Model file for the job. Use its own axes, mm. Face numbers are marked on the shaded views. A direction names the side the tool comes from. Coordinates: 2 decimals unless noted, no trailing zeros. Order: outer loops, then holes, each group sorted by start corner. A loop starts at its lowest first (then second) coordinate and runs counter-clockwise, first axis right, second up.
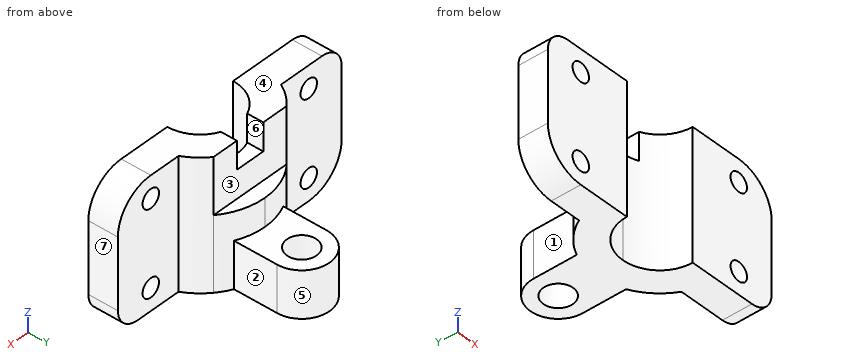
from build123d import *

# Parameters (mm, degrees)
EXTRUDE_1_DEPTH     = 70
CUT_EXTRUDE_2_DEPTH = 30
SKETCH_5_W          = 16
SKETCH_5_H          = 15
CUT_EXTRUDE_3_DEPTH = 102.257098517
EXTRUDE_START       = -25
SKETCH_6_R          = 8
EXTRUDE_2_DEPTH     = 25
SKETCH_7_R          = 5
CUT_EXTRUDE_4_DEPTH = 112.534747949
FILLET_1_R          = 20
FILLET_2_R          = 12


with BuildPart() as part:
    # Sketch 1 → Extrude 1 (new body)
    with BuildSketch(Plane.XY):
        with BuildLine():
            ThreePointArc((-20, 0), (-14.142135624, 14.142135624), (0, 20))
            Line((0, 20), (0, 27))
            Line((0, 27), (-22.271057451, 27))
            ThreePointArc((-22.271057451, 27), (-27.26050724, 21.951417836), (-31.128764833, 16))
            Line((-31.128764833, 16), (-68, 16))
            Line((-68, 16), (-68, 0))
            Line((-68, 0), (-20, 0))
        make_face()
        with BuildLine():
            Line((0, 27), (0, 20))
            ThreePointArc((0, 20), (14.142135624, 14.142135624), (20, 0))
            Line((20, 0), (68, 0))
            Line((68, 0), (68, 16))
            Line((68, 16), (31.128764833, 16))
            ThreePointArc((31.128764833, 16), (27.26050724, 21.951417836), (22.271057451, 27))
            Line((22.271057451, 27), (0, 27))
        make_face()
        with BuildLine():
            Line((-22.271057451, 27), (0, 27))
            Line((0, 27), (0, 35))
            ThreePointArc((0, 35), (-11.832159566, 32.939338184), (-22.271057451, 27))
        make_face()
        with BuildLine():
            Line((0, 35), (0, 27))
            Line((0, 27), (22.271057451, 27))
            ThreePointArc((22.271057451, 27), (11.832159566, 32.939338184), (0, 35))
        make_face()
    extrude(amount=-EXTRUDE_1_DEPTH)

    # Sketch 1_13 → Cut-Extrude 2 (cut)
    with BuildSketch(Plane.XY):
        with BuildLine():
            Line((-22.271057451, 27), (0, 27))
            Line((0, 27), (0, 35))
            ThreePointArc((0, 35), (-11.832159566, 32.939338184), (-22.271057451, 27))
        make_face()
        with BuildLine():
            Line((0, 35), (0, 27))
            Line((0, 27), (22.271057451, 27))
            ThreePointArc((22.271057451, 27), (11.832159566, 32.939338184), (0, 35))
        make_face()
    extrude(amount=-CUT_EXTRUDE_2_DEPTH, mode=Mode.SUBTRACT)

    # Sketch 5 → Cut-Extrude 3 (cut, through all)
    with BuildSketch(Plane(origin=(0, 27, 0), x_dir=(1, 0, 0), z_dir=(0, 1, 0))):
        with Locations((0, 7.5)):
            Rectangle(SKETCH_5_W, SKETCH_5_H)
    extrude(amount=-CUT_EXTRUDE_3_DEPTH, mode=Mode.SUBTRACT)

    # Sketch 6 → Extrude 2 (add)
    with BuildSketch(Plane(origin=(0, 0, -70), x_dir=(-1, 0, 0), z_dir=(0, 0, -1)).offset(EXTRUDE_START)):
        with BuildLine():
            Line((-15, 31.622776602), (-15, 55))
            ThreePointArc((-15, 55), (0, 70), (15, 55))
            Line((15, 55), (15, 31.622776602))
            ThreePointArc((15, 31.622776602), (0, 35), (-15, 31.622776602))
        make_face()
        with Locations((0, 55)):
            Circle(SKETCH_6_R, mode=Mode.SUBTRACT)
    extrude(amount=EXTRUDE_2_DEPTH)

    # Sketch 7 → Cut-Extrude 4 (cut, through all)
    with BuildSketch(Plane(origin=(0, 16, 0), x_dir=(1, 0, 0), z_dir=(0, 1, 0))):
        with Locations(Location((-48, 12, 0), (0, 0, 180))):
            Circle(SKETCH_7_R)
        with Locations((-48, 58)):
            Circle(SKETCH_7_R)
        with Locations(Location((48, 58, 0), (0, 0, 180))):
            Circle(SKETCH_7_R)
        with Locations((48, 12)):
            Circle(SKETCH_7_R)
    extrude(amount=-CUT_EXTRUDE_4_DEPTH, mode=Mode.SUBTRACT)

    # Fillet 1
    fillet_1_edges = [part.edges().sort_by_distance(p)[0] for p in [
        (68, 8, 0),
        (-68, 8, -70),
    ]]
    fillet(fillet_1_edges, radius=FILLET_1_R)

    # Fillet 2
    fillet_2_edges = [part.edges().sort_by_distance(p)[0] for p in [
        (-68, 8, 0),
        (68, 8, -70),
    ]]
    fillet(fillet_2_edges, radius=FILLET_2_R)


solid = part.part
Q1. Cut at B-B, the plane y = 24.5. List the corners of the cut face in (x, z) (3 decimals).
Established:
outline: (-24.995, -70) - (24.995, -70) - (24.995, 0) - (8, 0) - (8, -15) - (-8, -15) - (-8, 0) - (-24.995, 0) - close
Q2. Drop flat-ended pins along their axis: P1, Ø13, axis at x = 48, z = -12, coming from the +Y side; P2, Ø8, axis at x = -11, z = -29.5, coming from the +Y side; P3, Ø9, axis at x = 4, z = -9.5, coming from the +Y side; P4, Ø2, axis at x = -23.5, z = -26, coming from the -Y side. Give the stop position or say it passes through.
Established:
P1: stops at y = 16
P2: stops at y = 34.29
P3: stops at y = 27
P4: stops at y = 0
Q3. Cut at A-A, the plane y = 52. List the corners of the cut face in (x, z).
Established:
outline: (-15, -70) - (-7.42, -70) - (-7.42, -45) - (-15, -45) - close; (7.42, -70) - (15, -70) - (15, -45) - (7.42, -45) - close
Q4. Cut at D-D, the plane x = -25.5. List the corners of the cut face in (y, z), plus the area to 3 significant figures.
Established:
outline: (0, -70) - (23.97, -70) - (23.97, 0) - (0, 0) - close
area: 1,680 mm2
Q5. Mould opens along X. For the marked faces 4, 5, 6 and 7 say: pulls with the +X half, pulls with the -X half, needs draft (parallel to the pull), parting line crosses it, or undercut.
Established:
face 4: needs draft
face 5: parting line crosses it
face 6: undercut
face 7: pulls with the +X half
Q6. Cut at C-C, the plane x = 27. List the corners of the cut face in (y, z), plus the area to 3 significant figures.
Established:
outline: (0, -70) - (22.27, -70) - (22.27, 0) - (0, 0) - close
area: 1,560 mm2
Q7. Probe line 1 (Z direction, x = 48, y = 3.5); line 2 (Z direction, x = 8, y = 35.5); line 3 (Y direction, x = -38, z = -14.5). List the from-to ranges inside material, lowest first.
Established:
line 1: z = -70 to -63, -53 to -17, -7 to 0
line 2: z = -70 to -45
line 3: y = 0 to 16
Q8. Which spindle directions (+Z, -Z, +X, -X, +Y, -Y) get a long thin tool onto all of the face, cutting with end or side? Do the marked faces 1, 2 and 3. Say none if no direction does.
Established:
face 1: +Z, -Z, -X, +Y
face 2: +Z, -Z, +X, +Y
face 3: +Z, +X, -X, +Y
